```python
from build123d import *

# Parameters (mm, degrees)
SM_BASE_FLANGE_1_DEPTH = 670
SKETCH_2_W             = 20.2
SKETCH_2_H             = 3.1
CUT_EXTRUDE_1_DEPTH    = 10
SKETCH_4_W             = 20.2
SKETCH_4_H             = 3.1
CUT_EXTRUDE_3_DEPTH    = 10


# Sheet-metal steps are written as plain solids
with BuildPart() as part:
    # Sketch 1 → Базовая кромка1 (new body)
    with BuildSketch(Plane(origin=(0, 0, 0), x_dir=(1, 0, 0), z_dir=(0, 1, 0))):
        with BuildLine():
            Line((-31.146330545, 0), (-53.046330545, 0))
            ThreePointArc((-53.046330545, 0), (-55.238361567, -0.907968978), (-56.146330545, -3.1))
            Line((-56.146330545, -3.1), (-56.146330545, -26.9))
            ThreePointArc((-56.146330545, -26.9), (-55.238361567, -29.092031022), (-53.046330545, -30))
            Line((-53.046330545, -30), (440.753669455, -30))
            ThreePointArc((440.753669455, -30), (442.945700477, -29.092031022), (443.853669455, -26.9))
            Line((443.853669455, -26.9), (443.853669455, -3.1))
            ThreePointArc((443.853669455, -3.1), (442.945700477, -0.907968978), (440.753669455, 0))
            Line((440.753669455, 0), (418.853669455, 0))
            Line((418.853669455, 0), (418.853669455, -2))
            Line((418.853669455, -2), (440.753669455, -2))
            ThreePointArc((440.753669455, -2), (441.531486914, -2.322182541), (441.853669455, -3.1))
            Line((441.853669455, -3.1), (441.853669455, -26.9))
            ThreePointArc((441.853669455, -26.9), (441.531486914, -27.677817459), (440.753669455, -28))
            Line((440.753669455, -28), (-53.046330545, -28))
            ThreePointArc((-53.046330545, -28), (-53.824148004, -27.677817459), (-54.146330545, -26.9))
            Line((-54.146330545, -26.9), (-54.146330545, -3.1))
            ThreePointArc((-54.146330545, -3.1), (-53.824148004, -2.322182541), (-53.046330545, -2))
            Line((-53.046330545, -2), (-31.146330545, -2))
            Line((-31.146330545, -2), (-31.146330545, 0))
        make_face()
    extrude(amount=SM_BASE_FLANGE_1_DEPTH)

    # Эскиз2 → Вырез-Вытянуть1 (cut)
    with BuildSketch(Plane.XY.offset(30)):
        with Locations((53.853669455, 1.55)):
            Rectangle(SKETCH_2_W, SKETCH_2_H)
        with Locations((333.853669455, 1.55)):
            Rectangle(SKETCH_2_W, SKETCH_2_H)
    extrude(amount=-CUT_EXTRUDE_1_DEPTH, mode=Mode.SUBTRACT)

    # Эскиз4 → Вырез-Вытянуть3 (cut)
    with BuildSketch(Plane.XY.offset(30)):
        with Locations((53.853669455, 668.45)):
            Rectangle(SKETCH_4_W, SKETCH_4_H)
        with Locations((333.853669455, 668.45)):
            Rectangle(SKETCH_4_W, SKETCH_4_H)
    extrude(amount=-CUT_EXTRUDE_3_DEPTH, mode=Mode.SUBTRACT)


solid = part.part
```
The listing builds one solid part. Answer for the finished solid, in the listing's coordinates (mm). A direction names the side the tool comes from. Coordinates: 2 decimals unless noted, no trailing zeros. Write each loop counter-clockwise with the first axis right and the second up, starting at its lowest first coordinate (ties: lowest second). Pieces come first, ordered by that corner, then holes. Notation, with made-up numbers: (12.25, 58) - (67.25, 58) arc R20 cw to (67.25, 66) - close; hole circle Ø8 at (-13, 2.5). An arc over 180 degrees is marked (long way). Return JSON: item names as keys, results as strings. Group by question number.
1. A cutting plane is placed at B-B, the plane y = 111.5. Determine the outline of the cut face in (x, z), plus the area to 3 significant figures.
2. Straight lines are drawn through the part: L1, parallel to X at y = 361.5, z = 25.5; L2, parallel to X at y = 530, z = 27; L3, parallel to Z at x = 310, y = 398. For each, find the intervals that lie inside material, in ascending order.
3. Which of the six approach directions +Z, -Z, +X, -X, +Y, -Y give full straight-line access (tool end or side, diameter ignored) to faces 4 (the flat face through (-42, 330, 2)), 5 (the flat face through (-24.9, 0, 28.3))?
4. Given pin 1 (1.6 mm diameter, centred on y = 318, z = 0.5, fed in from +X); pin 2 (12 mm diameter, centred on x = 97, y = 90, fed in from -Z); pin 3 (0.6 mm diameter, centred on y = 455, z = 1, fed in from -X); pin 4 (12 mm diameter, centred on x = 34, z = 18.5, fed in from +Y), each flat-ended and moving along its own axis, determine where each tip first touches the part or whether it passes through.
5. Determine the mould class of faces 1 (the flat face through (430, 330, 0)), 2 (the flat face through (430, 330, 2)), 3 (the flat face through (401.1, 670, 28.3)) for opening direction Z: released by +Z, released by -Z, zero draft, split by the parting line, or undercut.
6. A cutting plane is placed at C-C, the plane x = -18. Determine the outline of the cut face in (y, z), plus the area to 3 significant figures.
7. A cutting plane is placed at A-A, the plane z = 17.5. Determine the outline of the cut face in (x, y).
Ans:
{
 "1": {"outline": "(-56.15, 3.1) arc R3.1 ccw to (-53.05, 0) - (-31.15, 0) - (-31.15, 2) - (-53.05, 2) arc R1.1 cw to (-54.15, 3.1) - (-54.15, 26.9) arc R1.1 cw to (-53.05, 28) - (440.75, 28) arc R1.1 cw to (441.85, 26.9) - (441.85, 3.1) arc R1.1 cw to (440.75, 2) - (418.85, 2) - (418.85, 0) - (440.75, 0) arc R3.1 ccw to (443.85, 3.1) - (443.85, 26.9) arc R3.1 ccw to (440.75, 30) - (-53.05, 30) arc R3.1 ccw to (-56.15, 26.9) - close", "area": "1,200 mm²"},
 "2": {"L1": "-56.15 to -54.15, 441.85 to 443.85", "L2": "-56.14 to -54.14, 441.85 to 443.85", "L3": "28 to 30"},
 "3": {"face 4": "+Y, -Y", "face 5": "+Z, -Z, +X, -X, -Y"},
 "4": {"pin 1": "x = 443.28", "pin 2": "z = 28", "pin 3": "x = -55.57", "pin 4": "through"},
 "5": {"face 1": "released by -Z", "face 2": "undercut", "face 3": "zero draft"},
 "6": {"outline": "(0, 28) - (670, 28) - (670, 30) - (0, 30) - close", "area": "1,340 mm²"},
 "7": {"outline": "(-56.15, 0) - (-54.15, 0) - (-54.15, 670) - (-56.15, 670) - close; (441.85, 0) - (443.85, 0) - (443.85, 670) - (441.85, 670) - close"}
}
